from build123d import *
from build123d.topology import SkipClean

# Parameters (mm, degrees)
SKETCH1_R           = 28.5
SKETCH1_R_2         = 15
BOSS_EXTRUDE1_DEPTH = 38
BOSS_EXTRUDE2_START = 16
SKETCH3_W           = 57
SKETCH3_H           = 84
SKETCH3_R           = 15
BOSS_EXTRUDE2_DEPTH = 16
BOSS_EXTRUDE3_DEPTH = 84
CUT_EXTRUDE1_DEPTH  = 28
SKETCH7_W           = 8
SKETCH7_H           = 7
CUT_EXTRUDE2_DEPTH  = 106.072593953


with BuildPart() as part:
    # Sketch1 → Boss-Extrude1 (new body)
    with BuildSketch(Plane(origin=(0, 0, 0), x_dir=(0, 0, -1), z_dir=(1, 0, 0))):
        Circle(SKETCH1_R)
        Circle(SKETCH1_R_2, mode=Mode.SUBTRACT)
    extrude(amount=BOSS_EXTRUDE1_DEPTH)

    # Sketch3 → Boss-Extrude2 (add)
    with SkipClean():  # the faces are left unmerged after this step: merging them gives an invalid solid
        with BuildSketch(Plane.ZY.offset(BOSS_EXTRUDE2_START)):
            Rectangle(SKETCH3_W, SKETCH3_H)
            Circle(SKETCH3_R, mode=Mode.SUBTRACT)
        extrude(amount=-BOSS_EXTRUDE2_DEPTH)

    # Sketch4 → Boss-Extrude3 (add)
    with SkipClean():  # the faces are left unmerged after this step: merging them gives an invalid solid
        with BuildSketch(Plane(origin=(0, 42, 0), x_dir=(1, 0, 0), z_dir=(0, 1, 0))):
            with BuildLine():
                Line((-16, 0), (-16, 28.5))
                Line((-16, 28.5), (-41.275105345, 18.629891095))
                ThreePointArc((-41.275105345, 18.629891095), (-50.515176458, 11.280467479), (-54, 0))
                Line((-54, 0), (-42, 0))
                ThreePointArc((-42, 0), (-34, 8), (-26, 0))
                Line((-26, 0), (-16, 0))
            make_face()
            with BuildLine():
                Line((-16, -28.5), (-16, 0))
                Line((-16, 0), (-26, 0))
                ThreePointArc((-26, 0), (-34, -8), (-42, 0))
                Line((-42, 0), (-54, 0))
                ThreePointArc((-54, 0), (-50.515176458, -11.280467479), (-41.275105345, -18.629891095))
                Line((-41.275105345, -18.629891095), (-16, -28.5))
            make_face()
        extrude(amount=-BOSS_EXTRUDE3_DEPTH)

    # Sketch5 → Cut-Extrude1 (cut, symmetric)
    with SkipClean():  # the faces are left unmerged after this step: merging them gives an invalid solid
        with BuildSketch(Plane(origin=(0, 0, 0), x_dir=(1, 0, 0), z_dir=(0, 1, 0))):
            with BuildLine():
                Line((-16, 28.5), (-41.275105345, 18.629891095))
                ThreePointArc((-41.275105345, 18.629891095), (-54, 0), (-41.275105345, -18.629891095))
                Line((-41.275105345, -18.629891095), (-16, -28.5))
                Line((-16, -28.5), (-16, 28.5))
            make_face()
        extrude(amount=CUT_EXTRUDE1_DEPTH, both=True, mode=Mode.SUBTRACT)

    # Sketch7 → Cut-Extrude2 (cut, through all)
    with SkipClean():  # the faces are left unmerged after this step: merging them gives an invalid solid
        with BuildSketch(Plane(origin=(38, 0, 0), x_dir=(0, 0, -1), z_dir=(1, 0, 0))):
            with Locations((0, 15)):
                Rectangle(SKETCH7_W, SKETCH7_H)
        extrude(amount=-CUT_EXTRUDE2_DEPTH, mode=Mode.SUBTRACT)
    add(part.part.scale(1), mode=Mode.REPLACE)  # the faces are merged on a copy


solid = part.part
Build history of the part. All positions in model axes, mm. A direction names the side the tool comes from. Give positions to 0.01 mm unless a question says otherwise; leave off trailing zeros. Order: outer loops, then holes, each group sorted by start corner. A loop starts at its lowest first (then second) coordinate and runs counter-clockwise, first axis right, second up. Notation, with made-up numbers: M -23.75,69.25 L 8.25,69.25 A15 cw 8.25,96.25 Z; hole C -22,72 d6. An arc over 180 degrees is marked long. Put each result on its own line as item: value.
Item 1: 3-axis set-ups, long thin cutter, end or side, ignore diameter. For faces 5 (the flat face through (0, 31, 0)), 6 (the cylindrical face through (18.734, -10.916, -26.327)), 7 (the flat face through (11, 16, -4)), 8 (the flat face through (-27, -28, 6)), 9 (the flat face through (38, -12, -12)): which of +Z, -Z, +X, -X, +Y, -Y reach the whole face in a straight line?
From the geometry:
face 5: +X, +Y
face 6: +X
face 7: +X, -X
face 8: +Z, -Z, -X
face 9: +Z, -Z, +X, +Y, -Y
Item 2: Slice it at B-B, the plane z = -13.5. Write the cut outline in (x, y), plus the area to 3 significant figures.
From the geometry:
outline: M -48.76,-42 L 0,-42 L 0,-25.1 L 38,-25.1 L 38,-6.54 L -16,-6.54 L -16,-28 L -48.76,-28 Z; M -48.76,28 L -16,28 L -16,6.54 L 38,6.54 L 38,25.1 L 0,25.1 L 0,42 L -48.76,42 Z
area: 3,460 mm2
Item 3: Slice it at D-D, the plane y = -23. Write the cut outline in (x, z), plus the area to 3 significant figures.
From the geometry:
outline: M -16,-28.5 L 0,-28.5 L 0,-16.83 L 38,-16.83 L 38,16.83 L 0,16.83 L 0,28.5 L -16,28.5 Z
area: 2,190 mm2
Item 4: Slice it at C-C, the plane x = -34. Write the cut outline in (y, z).
From the geometry:
outline: M -42,-21.47 L -28,-21.47 L -28,-8 L -42,-8 Z; M -42,8 L -28,8 L -28,21.47 L -42,21.47 Z; M 28,-21.47 L 42,-21.47 L 42,-8 L 28,-8 Z; M 28,8 L 42,8 L 42,21.47 L 28,21.47 Z
Item 5: Slice it at A-A, the plane x = 9. Write the cut outline in (y, z), plus the area to 3 significant figures.
From the geometry:
outline: C 0,0 d57; hole M 14.46,-4 L 18.5,-4 L 18.5,4 L 14.46,4 A15 ccw long Z
area: 1,820 mm2
Item 6: Two-plate mould, pull along Z, no slides. Class faces 1 (the flat face through (11, 18.5, 0)), 2 (the flat face through (-28.8, -34.9, 23.5)), 3 (the flat face through (-16, 13, -12)), 4 (the flat face through (11, 16, 4)): +Z half, -Z half, draft (parallel to the pull), parting line (faces both ways), or undercut.
From the geometry:
face 1: undercut
face 2: +Z half
face 3: draft
face 4: undercut
Item 7: Probe line 1 (Y direction, x = -10.5, z = 0); line 2 (Y direction, x = -19, z = 25.5); line 3 (Z direction, x = -6.5, y = 0). List the from-to ranges inside material, lowest first. Write a range as [from, to].
From the geometry:
line 1: y = [-42, -15], [18.5, 42]
line 2: y = [-42, -28], [28, 42]
line 3: z = [-28.5, -15], [15, 28.5]
Item 8: Flat gauge pins, fed straight in: pin 1 Ø5 at (y, z) = (-11.5, -7.5) entering from -X; pin 2 Ø4.5 at (x, y) = (2.5, 15.5) entering from +Z; pin 3 Ø1.5 at (x, y) = (19.5, -4.5) entering from +Z. Where does each tip first touch, or does it go through?
From the geometry:
pin 1: stops at x = -16
pin 2: stops at z = 25.23
pin 3: stops at z = 28.25
